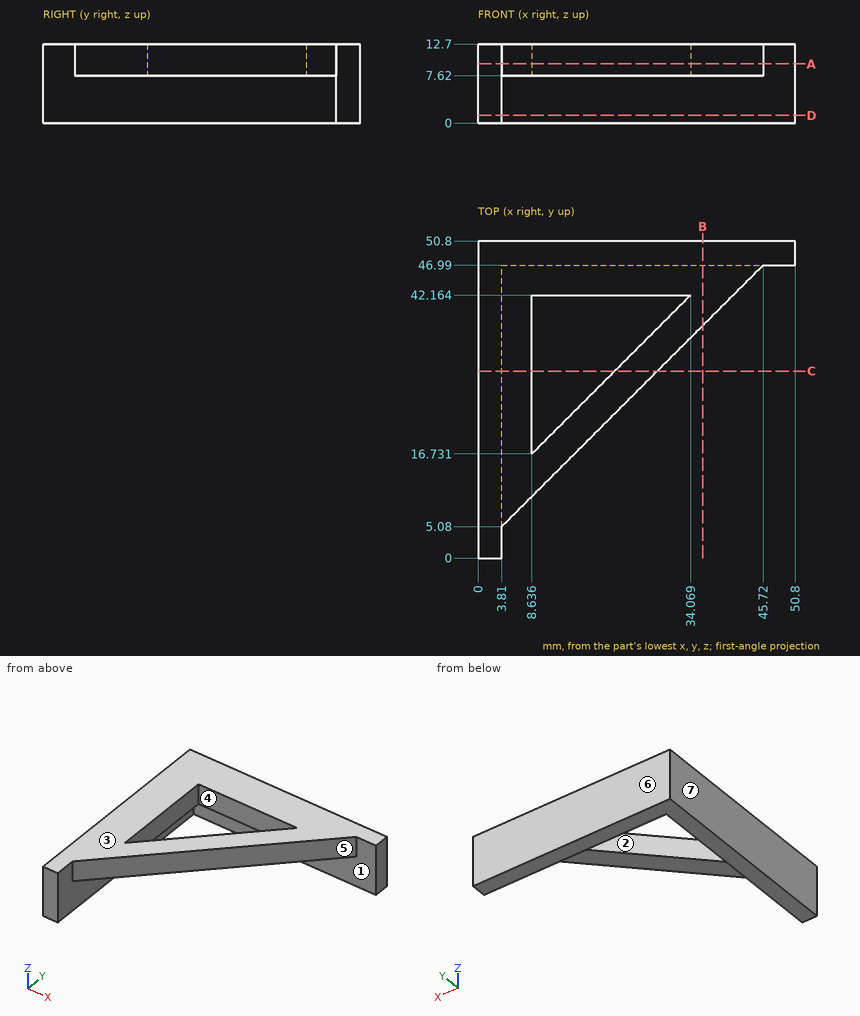
Part print with two shaded views. Sizes in mm from the minimum x, y, z corner. A direction names the side the tool comes from. Coordinates: 2 decimals unless noted, no trailing zeros. Write each loop counter-clockwise with the first axis right and the second up, starting at its lowest first coordinate (ties: lowest second). Pieces come first, ordered by that corner, then holes. Notation, with made-up numbers: (81, 12.25) - (128, 12.25) arc R15 ccw to (128, 34.25) - close; hole circle Ø9 at (-12.5, 35.25). An arc over 180 degrees is marked (long way). Use a Markdown table: item, result. Add a question column.
Item 1: Two-plate mould, pull along Y, no slides. Class the marked faces 4, 5, 6 and 7: pulls with the +Y half, pulls with the -Y half, needs draft (parallel to the pull), parting line crosses it, or undercut.
Item 2: Band-saw the part on C-C, the plane y = 30. Write the cut outline in (x, z) (3 decimals), and give its area (3 significant figures).
Item 3: Band-saw the part on A-A, the plane z = 9.5. Write the cut outline in (x, y).
Item 4: Drop flat-ended pins along their axis: pin 1 (12.5 mm diameter, centred on x = 21.5, y = 24, fed in from -Z); pin 2 (1 mm diameter, centred on x = 10.5, y = 39.5, fed in from -Z) (1 decimal); pin 3 (2.5 mm diameter, centred on x = 24.5, z = 10.5, fed in from -Y); pin 4 (4 mm diameter, centred on y = 28, z = 9.5, fed in from +X). Give the stop position or say it passes through.
Item 5: 3-axis set-ups, long thin cutter, end or side, ignore diameter. For the marked faces 1, 2 and 3: which of +Z, -Z, +X, -X, +Y, -Y reach the whole face in a straight line?
Item 6: Band-saw the part on D-D, the plane z = 1.25. Write the cut outline in (x, y), and give its area (3 significant figures).
Item 7: Drill centre lines: line 1 along X through (y, z) = (38.5, 4.75); line 2 along X through (y, z) = (22, 9.25) (3 decimals); line 3 along Y through (x, z) = (15, 5). Where is each one in solid material? Low to high.
Item 8: Band-saw the part on B-B, the plane x = 36. Write the cut outline in (y, z), and give its area (3 significant figures).
A:
| question | item | result |
|---|---|---|
| 1 | face 4 | undercut |
| 1 | face 5 | pulls with the -Y half |
| 1 | face 6 | pulls with the +Y half |
| 1 | face 7 | needs draft |
| 2 | outline | (0, 0) - (3.81, 0) - (3.81, 7.62) - (8.636, 7.62) - (8.636, 12.7) - (0, 12.7) - close; (21.905, 7.62) - (28.73, 7.62) - (28.73, 12.7) - (21.905, 12.7) - close |
| 2 | area | 108 mm² |
| 3 | outline | (0, 0) - (3.81, 0) - (3.81, 5.08) - (45.72, 46.99) - (50.8, 46.99) - (50.8, 50.8) - (0, 50.8) - close; hole (8.64, 16.73) - (34.07, 42.16) - (8.64, 42.16) - close |
| 4 | pin 1 | stops at z = 7.62 |
| 4 | pin 2 | passes through |
| 4 | pin 3 | stops at y = 24.52 |
| 4 | pin 4 | stops at x = 28.73 |
| 5 | face 1 | -Z, +X, -Y |
| 5 | face 2 | +Z, -Z |
| 5 | face 3 | +Z, +X, -X, +Y, -Y |
| 6 | outline | (0, 0) - (3.81, 0) - (3.81, 46.99) - (50.8, 46.99) - (50.8, 50.8) - (0, 50.8) - close |
| 6 | area | 373 mm² |
| 7 | line 1 | x = 0 to 3.81 |
| 7 | line 2 | x = 0 to 8.636, 13.905 to 20.73 |
| 7 | line 3 | y = 46.99 to 50.8 |
| 8 | outline | (37.27, 7.62) - (46.99, 7.62) - (46.99, 0) - (50.8, 0) - (50.8, 12.7) - (37.27, 12.7) - close |
| 8 | area | 97.8 mm² |
